from build123d import *

# Parameters (mm, degrees)
SKETCH1_W           = 6
SKETCH1_H           = 66
SKETCH1_W_2         = 44
SKETCH1_H_2         = 6
BOSS_EXTRUDE1_DEPTH = 50
FILLET1_R           = 25
SKETCH3_R           = 1.6
SKETCH3_R_2         = 4
CUT_EXTRUDE2_DEPTH  = 88.527138649
SKETCH4_R           = 1.55
CUT_EXTRUDE3_DEPTH  = 88.407093534


with BuildPart() as part:
    # Sketch1 → Boss-Extrude1 (new body)
    with BuildSketch(Plane.XY):
        with Locations((-25, 12)):
            Rectangle(SKETCH1_W, SKETCH1_H)
        with Locations((0, -24)):
            Rectangle(SKETCH1_W_2, SKETCH1_H_2)
        with Locations((-25, -24)):
            Rectangle(SKETCH1_W, SKETCH1_H_2)
        with Locations((25, -24)):
            Rectangle(SKETCH1_W, SKETCH1_H_2)
        with Locations((25, 12)):
            Rectangle(SKETCH1_W, SKETCH1_H)
    extrude(amount=BOSS_EXTRUDE1_DEPTH)

    # Fillet1
    fillet1_edges = [part.edges().sort_by_distance(p)[0] for p in [
        (-25, 45, 50),
        (-25, 45, 0),
        (25, 45, 0),
        (25, 45, 50),
    ]]
    fillet(fillet1_edges, radius=FILLET1_R - 0.0001)  # a hair under: the kernel refuses the full size

    # Sketch3 → Cut-Extrude2 (cut, through all)
    with BuildSketch(Plane(origin=(28, 0, 0), x_dir=(0, 0, -1), z_dir=(1, 0, 0))):
        with Locations(Location((-12.941245902, 30, 0), (0, 0, 90))):
            Circle(SKETCH3_R)
        with Locations(Location((-24.941245902, 30, 0), (0, 0, 90))):
            Circle(SKETCH3_R_2)
    extrude(amount=-CUT_EXTRUDE2_DEPTH, mode=Mode.SUBTRACT)

    # Sketch4 → Cut-Extrude3 (cut, through all)
    with BuildSketch(Plane(origin=(0, -21, 0), x_dir=(1, 0, 0), z_dir=(0, 1, 0))):
        with Locations(Location((-14.142135624, -38, 0), (0, 0, 270))):
            Circle(SKETCH4_R)
        with Locations(Location((14.142135624, -38, 0), (0, 0, 270))):
            Circle(SKETCH4_R)
        with Locations(Location((0, -13, 0), (0, 0, 270))):
            Circle(SKETCH4_R)
    extrude(amount=-CUT_EXTRUDE3_DEPTH, mode=Mode.SUBTRACT)


solid = part.part
Part model, mm, in its own coordinate system. A direction names the side the tool comes from. Coordinates: 2 decimals unless noted, no trailing zeros. Order: outer loops, then holes, each group sorted by start corner. A loop starts at its lowest first (then second) coordinate and runs counter-clockwise, first axis right, second up.
(1) Slice it at A-A, the plane x = 0. Write the cut outline in (y, z), and give its area (3 significant figures).
Check sheet entries:
outline: (-27, 0) - (-21, 0) - (-21, 11.45) - (-27, 11.45) - close; (-27, 14.55) - (-21, 14.55) - (-21, 50) - (-27, 50) - close
area: 281 mm2
(2) Probe L1, parallel to X at y = -22.55, z = 38; L2, parallel to Z at x = 25.2, y = 30; L3, parallel to X at y = 29, z = 47.5. List the from-to ranges inside material, lowest first.
Check sheet entries:
L1: x = -28 to -15.69, -12.59 to 12.59, 15.69 to 28
L2: z = 2.09 to 11.34, 14.54 to 20.94, 28.94 to 47.91
L3: x = -28 to -22, 22 to 28
(3) Slice it at D-D, the plane x = 9. Write the cut outline in (y, z), and give its area (3 significant figures).
Check sheet entries:
outline: (-27, 0) - (-21, 0) - (-21, 50) - (-27, 50) - close
area: 300 mm2
(4) Tool access for faces 5 (the face through (22, 12, 25)), 6 (the face through (-28, 10, 25)): list every direction of +Z, -Z, +X, -X, +Y, -Y with a clear straight run to the whole face (end or side of a thin tool).
Check sheet entries:
face 5: +Z, -Z, +Y
face 6: +Z, -Z, -X, +Y, -Y
(5) Slice it at B-B, the plane y = 10. Write the cut outline in (x, z), and give its area (3 significant figures).
Check sheet entries:
outline: (-28, 0) - (-22, 0) - (-22, 50) - (-28, 50) - close; (22, 0) - (28, 0) - (28, 50) - (22, 50) - close
area: 600 mm2
(6) Pin check, flat tips, straight feed: pin 1 Ø1.9 at (x, z) = (-14.14, 38) entering from +Y; pin 2 Ø4 at (x, y) = (22, 37.5) entering from -Z; pin 3 Ø1 at (x, z) = (0.5, 24.5) entering from +Y. Stop position of each tip, or through.
Check sheet entries:
pin 1: passes through
pin 2: stops at z = 5.38
pin 3: stops at y = -21
(7) Slice it at C-C, the plane z = 38. Write the cut outline in (x, y).
Check sheet entries:
outline: (-28, -27) - (-15.69, -27) - (-15.69, -21) - (-22, -21) - (-22, 41.35) - (-28, 41.35) - close; (-12.59, -27) - (12.59, -27) - (12.59, -21) - (-12.59, -21) - close; (15.69, -27) - (28, -27) - (28, 41.35) - (22, 41.35) - (22, -21) - (15.69, -21) - close
(8) Pull direction Z, two halves, no side cores. Call faces 1 (the face through (-22, 12, 25)), 2 (the face through (12.77, -23.96, 38.72)), 3 (the face through (0, -23, 50)), 4 (the face through (0, -23, 0)): pulls with the +Z half, pulls with the -Z half, needs draft (parallel to the pull), parting line crosses it, or undercut.
Check sheet entries:
face 1: needs draft
face 2: undercut
face 3: pulls with the +Z half
face 4: pulls with the -Z half
